```python
from build123d import *

# Parameters (mm, degrees)
F0_W      = 80
F0_H      = 10
F1_DEPTH  = 10
F2_W      = 4
F2_H      = 4
F3_DEPTH  = 2
F4_W      = 4
F4_H      = 4
F5_DEPTH  = 2
F6_T      = -2.5
F7_W      = 2.5
F7_H      = 7.5
F8_DEPTH  = 7.5
F9_R      = 1.65
F10_DEPTH = 41.25


with BuildPart() as f1:
    # F0 (on Top) → F1 (new body)
    with BuildSketch(Plane.XY):
        Rectangle(F0_W, F0_H)
    extrude(amount=F1_DEPTH)

    # F2 (on face) → F3 (join)
    with BuildSketch(Plane.YZ.offset(40)):
        with Locations((0, 5)):
            Rectangle(F2_W, F2_H)
    extrude(amount=F3_DEPTH)

    # F4 (on face) → F5 (join)
    with BuildSketch(Plane(origin=(-40, 0, 0), x_dir=(0, -1, 0), z_dir=(-1, 0, 0))):
        with Locations((0, 5)):
            Rectangle(F4_W, F4_H)
    extrude(amount=F5_DEPTH)

    # F6
    f6_openings = [f1.faces().sort_by_distance(p)[0] for p in [
        (0, -5, 5),
        (0, 0, 10),
    ]]
    offset(amount=F6_T, openings=f6_openings, kind=Kind.INTERSECTION)

    # F7 (on face) → F8 (join, through all)
    with BuildSketch(Plane.XY.offset(2.5)):
        with Locations((-19.375, -1.25)):
            Rectangle(F7_W, F7_H)
        with Locations((0, -1.25)):
            Rectangle(F7_W, F7_H)
        with Locations((19.375, -1.25)):
            Rectangle(F7_W, F7_H)
    extrude(amount=F8_DEPTH)

    # F9 (on face) → F10 (cut, through all)
    with BuildSketch(Plane(origin=(-20.625, 0, 0), x_dir=(0, -1, 0), z_dir=(-1, 0, 0))):
        with Locations((1.25, 6.25)):
            Circle(F9_R)
    extrude(amount=-F10_DEPTH, mode=Mode.SUBTRACT)


solid = f1.part
```
For this review, take the finished solid that the model builds, in its own axes (mm). A direction names the side the tool comes from. Round coordinates to 2 decimals unless told otherwise and drop trailing zeros. Write each loop counter-clockwise with the first axis right and the second up, starting at its lowest first coordinate (ties: lowest second). Pieces come first, ordered by that corner, then holes. Notation, with made-up numbers: M -16,67 L 0,67 A23 ccw 0,82 Z; hole C -18,85.25 d2. An arc over 180 degrees is marked long. One line per item, written item: value. Start each with the question number.
(1) We need section D-D (y = 4). Give the boundary of the cut face in (x, z), and give its area (3 significant figures).
(2) We need section B-B (x = -7). Give the boundary of the cut face in (y, z).
(3) We need section C-C (y = -1.25). Count the separate pieces of the cut face and the enclosed holes in it, and give its area (3 significant figures).
(4) Wall thickness on line 1 (X direction, y = -3, z = 6.5) (3 decimals); line 2 (X direction, y = 0, z = 3.5) (3 decimals); line 3 (Z direction, x = -0.7, y = -1.25): over which ranges is each line inside the solid? List them lowest first.
(5) The part is to be moulded in two halves that separate along X. For faces 1 (the flat face through (29, -1, 2.5)), 2 (the flat face through (42, 0, 5)), 3 (the flat face through (-41, 2, 5)), say which applies: released by +X, released by -X, zero draft, split by the parting line, or undercut.
(6) Machinability: for faces 4 (the flat face through (41, 0, 3)), 5 (the cylindrical face through (-19.39, -0.89, 4.64)), 6 (the flat face through (-41, -2, 5)), 7 (the flat face through (-29, -1, 2.5)), which of the approach directions +Z, -Z, +X, -X, +Y, -Y give a long, thin tool a straight path to every point of the face, cutting with its end or side? Answer none if there is none.
(7) We need section A-A (z = 8.75). Give the boundary of the cut face in (x, y) (3 decimals), and give its area (3 significant figures).
(8) Insertion check: pin 1 (6 mm diameter, centred on x = 5, z = 8.5, fed in from -Y); pin 2 (1.6 mm diameter, centred on x = 41.5, z = 6, fed in from -Y); pin 3 (2 mm diameter, centred on x = 7, y = -0.5, fed in from -Z); pin 4 (2 mm diameter, centred on x = 41.5, z = 4.5, fed in from +Y). Each pin has a flat end and moves straight along its axis. Give the tip position at first contact, or say it passes through.
Result:
1. outline: M -40,0 L 40,0 L 40,10 L -40,10 Z
1. area: 800 mm²
2. outline: M -5,0 L 5,0 L 5,10 L 2.5,10 L 2.5,2.5 L -5,2.5 Z
3. separate pieces: 4
3. enclosed holes: 0
3. area: 285 mm²
4. line 1: -40 to -37.5, -20.625 to -18.125, -1.25 to 1.25, 18.125 to 20.625, 37.5 to 40
4. line 2: -42 to -37.5, -20.625 to -18.125, -1.25 to 1.25, 18.125 to 20.625, 37.5 to 42
4. line 3: 0 to 4.6, 7.9 to 10
5. face 1: undercut
5. face 2: released by +X
5. face 3: zero draft
6. face 4: -Z, +X, +Y, -Y
6. face 5: none
6. face 6: +Z, -Z, -X, -Y
6. face 7: +Z, -Y
7. outline: M -40,-5 L -37.5,-5 L -37.5,2.5 L -20.625,2.5 L -20.625,-5 L -18.125,-5 L -18.125,2.5 L -1.25,2.5 L -1.25,-5 L 1.25,-5 L 1.25,2.5 L 18.125,2.5 L 18.125,-5 L 20.625,-5 L 20.625,2.5 L 37.5,2.5 L 37.5,-5 L 40,-5 L 40,5 L -40,5 Z
7. area: 294 mm²
8. pin 1: y = 2.5
8. pin 2: y = -2
8. pin 3: z = 0
8. pin 4: y = 2
